Autodesk Inventor part; units mm, degrees
ref_plane "YZ Plane" through (0, 0, 0) normal (1, 0, 0) x (0, 1, 0)
ref_plane "XZ Plane" through (0, 0, 0) normal (0, 1, 0) x (-1, 0, 0)
ref_plane "XY Plane" through (0, 0, 0) normal (0, 0, 1) x (1, 0, 0)
sketch "Szkic1" plane through (0, 0, 0) normal (0, 1, 0) x (-1, 0, 0)
  circle A0 centre (0, 0) radius 10
  dimension "d0" = 20
extrude "Wyciągnięcie proste1" add sketch "Szkic1" along normal mid plane 30
sketch "Szkic2" plane through (0, 15, 0) normal (0, 1, 0) x (1, 0, 0)
  circle A0 centre (0, 0) radius 10
  circle A1 centre (0, 0) radius 7.5
  dimension "d3" = 15
extrude "Wyciągnięcie proste2" add sketch "Szkic2" along normal blind 15 contours A1
sketch "Szkic3" plane through (0, 30, 0) normal (0, 1, 0) x (1, 0, 0)
  circle A0 centre (0, 0) radius 7.5
  circle A1 centre (0, 0) radius 10
  dimension "d6" = 20
extrude "Wyciągnięcie proste3" add sketch "Szkic3" along normal blind 5 contours A0 | A1
mirror "Odbicie lustrzane1" about plane through (0, 0, 0) normal (0, 1, 0) of "Wyciągnięcie proste3", "Wyciągnięcie proste2"
sketch "Szkic4" plane through (0, 0, 0) normal (1, 0, 0) x (0, 1, 0)
  point P0 (0, 0)
properties part number "RevolvingConnector1" material "Aluminium 6061"
Can you work these out from the model? Positions are in its coordinate system, mm. A direction names the side the tool comes from. Round coordinates to 2 decimals unless told otherwise and drop trailing zeros. Loops run counter-clockwise (first coordinate to the right, second up) from the corner with the lowest first, then second, coordinate; pieces in that order, holes last. Notation, with made-up numbers: (79.25, 5) - (93.25, 5) arc R20 ccw to (93.25, 37) - close; hole circle Ø4 at (0, -18). An arc over 180 degrees is marked (long way). Use CSV: the item, a comma, the result in double quotes. Start each with the question number.
1) We'd pull the mould along Y, two halves only. Please class faces 1 (the flat face through (0, 35, 0)), 2 (the flat face through (-4, -15, 7)), 3 (the cylindrical face through (-2.17, 32.47, -9.76)): released by +Y, released by -Y, zero draft, split by the parting line, or undercut.
2) If we section it at D-D on y = -8: Write out the boundary of the cut face in (x, z), plus the area to 3 significant figures.
3) If we section it at A-A on x = 0: Write out the boundary of the cut face in (y, z), plus the area to 3 significant figures.
4) Please list where these lines run through material, in increasing order: probe 1 along Y at (x, z) = (5.75, -6.5); probe 2 along Z at (x, y) = (0.5, -7); probe 3 along X at (y, z) = (2, 0.25). Write a range as [from, to].
5) For faces 4 (the cylindrical face through (-7.493, 22.395, 0.33)), 5 (the cylindrical face through (-2.17, -32.47, 9.76)), which set-ups out of +Z, -Z, +X, -X, +Y, -Y let a thin tool reach every point of the face, with its end or its side?
6) If we section it at B-B on z = -6: Write out the boundary of the cut face in (x, y).
7) For pin 1 Ø2 at (x, y) = (5, 22) entering from -Z; pin 2 Ø1 at (y, z) = (10, -4) entering from +X; pin 3 Ø12 at (x, y) = (-1, -25) entering from +Z; pin 4 Ø6 at (y, z) = (9, -5) entering from +X, each with a flat end and sliding along its axis, tell me the tip position at first contact or that it passes through.
8) If we section it at C-C on y = -28: Write out the boundary of the cut face in (x, z).
Geometry results:
1,face 1,"released by +Y"
1,face 2,"undercut"
1,face 3,"zero draft"
2,outline,"circle Ø20 at (0, 0)"
2,area,"314 mm2"
3,outline,"(-35, -10) - (-30, -10) - (-30, -7.5) - (-15, -7.5) - (-15, -10) - (15, -10) - (15, -7.5) - (30, -7.5) - (30, -10) - (35, -10) - (35, 10) - (30, 10) - (30, 7.5) - (15, 7.5) - (15, 10) - (-15, 10) - (-15, 7.5) - (-30, 7.5) - (-30, 10) - (-35, 10) - close"
3,area,"1,250 mm2"
4,probe 1,"y = [-35, -30], [-15, 15], [30, 35]"
4,probe 2,"z = [-9.99, 9.99]"
4,probe 3,"x = [-10, 10]"
5,face 4,"none"
5,face 5,"+Y, -Y"
6,outline,"(-8, -35) - (8, -35) - (8, -30) - (4.5, -30) - (4.5, -15) - (8, -15) - (8, 15) - (4.5, 15) - (4.5, 30) - (8, 30) - (8, 35) - (-8, 35) - (-8, 30) - (-4.5, 30) - (-4.5, 15) - (-8, 15) - (-8, -15) - (-4.5, -15) - (-4.5, -30) - (-8, -30) - close"
7,pin 1,"stops at z = -6.34"
7,pin 2,"stops at x = 9.37"
7,pin 3,"stops at z = 10"
7,pin 4,"stops at x = 9.8"
8,outline,"circle Ø15 at (0, 0)"
